Here's how the part is built. I have some questions about the finished solid (model axes, mm). A direction names the side the tool comes from. Round coordinates to 2 decimals unless told otherwise and drop trailing zeros. Put each result on its own line as item: value. Start each with the question number.
1. Suppose I cut it at A-A (x = 0). Count the separate pieces of the cut face and the enclosed holes in it, then the cut area to 3 significant figures.
2. For pin 1 (6 mm diameter, centred on x = -16, y = 17, fed in from -Z); pin 2 (1.5 mm diameter, centred on x = 1.5, z = -10, fed in from -Y); pin 3 (2.5 mm diameter, centred on x = -1.5, y = -0.5, fed in from -Z), each with a flat end and sliding along its axis, tell me the tip position at first contact or that it passes through.
3. We'd pull the mould along X, two halves only. Please class faces 4 (the face through (0, 0, 0)), 5 (the face through (-18.57, -0.65, -12.63)): +X half, -X half, draft (parallel to the pull), parting line (faces both ways), or undercut.
4. Which directions (+Z, -Z, +X, -X, +Y, -Y) give clear straight access to the entire face, cutting with the end or side of a thin tool? Please do faces 1 (the face through (-0.221, 19.686, -2.465)), 2 (the face through (0, -16, -5)), 3 (the face through (-11.547, -14.588, -1.479)).
5. I need wall thicknesses on probe 1 along Y at (x, z) = (8.5, -16); probe 2 along Y at (x, z) = (11, -2.25); probe 3 along Z at (x, y) = (-19, -9). Which ranges of each line are inside material? Lowest first, please. Write a range as from..to.
```python
from build123d import *

# Parameters (mm, degrees)
SKETCH_1_W                   = 25
SKETCH_1_H                   = 1
SKETCH_2_R                   = 22.55
EXTRUDE_1_DEPTH              = 10
HOLE_WIZARD_M3_1_D           = 3.4
HOLE_WIZARD_M3_1_DEPTH       = 11
HOLE_WIZARD_M3_1_CBORE_D     = 4.5
HOLE_WIZARD_M3_1_CBORE_DEPTH = 6
HOLE_WIZARD_1_D              = 8
HOLE_WIZARD_1_DEPTH          = 5
HOLE_WIZARD_1_CBORE_D        = 10.16
HOLE_WIZARD_1_CBORE_DEPTH    = 3
HOLE_WIZARD_M3_2_D           = 3.4
HOLE_WIZARD_M3_2_DEPTH       = 22
HOLE_WIZARD_M3_2_CBORE_D     = 6.1
HOLE_WIZARD_M3_2_CBORE_DEPTH = 3
CHAMFER_1_SIZE               = 1.05


with BuildPart() as part:
    # 草图1 → 旋转1 (revolve)
    with BuildSketch(Plane(origin=(0, 0, 0), x_dir=(1, 0, 0), z_dir=(0, 1, 0))):
        with Locations((12.5, 10.5)):
            Rectangle(SKETCH_1_W, SKETCH_1_H)
    revolve(axis=Axis((0, 0, -11), (0, 0, 1)))

    # 草图2 → 凸台-拉伸1 (add)
    with BuildSketch(Plane.XY.offset(-10)):
        Circle(SKETCH_2_R)
    extrude(amount=EXTRUDE_1_DEPTH)

    # 草图3 → 旋转2 (revolve)
    with BuildSketch(Plane(origin=(0, -14.722431864, 0), x_dir=(1, 0, 0), z_dir=(0, 1, 0))):
        Polygon((11.56, 22), (8.5, 22), (8.5, 11), (12.5, 11), (12.5, 12.5), (11.56, 12.5), align=None)
    revolve(axis=Axis((8.5, -14.722431864, -22), (0, 0, 1)))

    # 草图4 → 旋转3 (revolve)
    with BuildSketch(Plane(origin=(0, -14.722431864, 0), x_dir=(1, 0, 0), z_dir=(0, 1, 0))):
        Polygon((-5.44, 22), (-8.5, 22), (-8.5, 11), (-4.5, 11), (-4.5, 12.5), (-5.44, 12.5), align=None)
    revolve(axis=Axis((-8.5, -14.722431864, -22), (0, 0, 1)))

    # 草图5 → 旋转4 (revolve)
    with BuildSketch(Plane(origin=(0, 0, 0), x_dir=(1, 0, 0), z_dir=(0, 1, 0))):
        Polygon((-13.94, 22), (-17, 22), (-17, 11), (-13, 11), (-13, 12.5), (-13.94, 12.5), align=None)
    revolve(axis=Axis((-17, 0, -22), (0, 0, 1)))

    # 草图6 → 旋转5 (revolve)
    with BuildSketch(Plane(origin=(0, 14.722431864, 0), x_dir=(1, 0, 0), z_dir=(0, 1, 0))):
        Polygon((-5.44, 22), (-8.5, 22), (-8.5, 11), (-4.5, 11), (-4.5, 12.5), (-5.44, 12.5), align=None)
    revolve(axis=Axis((-8.5, 14.722431864, -22), (0, 0, 1)))

    # 草图7 → 旋转6 (revolve)
    with BuildSketch(Plane(origin=(0, 14.722431864, 0), x_dir=(1, 0, 0), z_dir=(0, 1, 0))):
        Polygon((11.56, 22), (8.5, 22), (8.5, 11), (12.5, 11), (12.5, 12.5), (11.56, 12.5), align=None)
    revolve(axis=Axis((8.5, 14.722431864, -22), (0, 0, 1)))

    # 草图8 → 旋转7 (revolve)
    with BuildSketch(Plane(origin=(0, 0, 0), x_dir=(1, 0, 0), z_dir=(0, 1, 0))):
        Polygon((20.06, 22), (17, 22), (17, 11), (21, 11), (21, 12.5), (20.06, 12.5), align=None)
    revolve(axis=Axis((17, 0, -22), (0, 0, 1)))

    # M3 六角头机械螺钉的柱形沉头孔1
    with Locations(Plane(origin=(0, 0, -11), x_dir=(-1, 0, 0), z_dir=(0, 0, -1))):
        with Locations((15.588457268, 9), (0, 18), (-15.588457268, 9), (-15.588457268, -9), (0, -18), (15.588457268, -9)):
            CounterBoreHole(HOLE_WIZARD_M3_1_D / 2, HOLE_WIZARD_M3_1_CBORE_D / 2, HOLE_WIZARD_M3_1_CBORE_DEPTH, depth=HOLE_WIZARD_M3_1_DEPTH)

    # 孔1
    with Locations(Plane(origin=(0, 0, -11), x_dir=(-1, 0, 0), z_dir=(0, 0, -1))):
        with Locations((0, 0)):
            CounterBoreHole(HOLE_WIZARD_1_D / 2, HOLE_WIZARD_1_CBORE_D / 2, HOLE_WIZARD_1_CBORE_DEPTH, depth=HOLE_WIZARD_1_DEPTH)

    # M3 六角头机械螺钉的柱形沉头孔2
    with Locations(Plane.XY):
        with Locations((8.5, -14.722431864), (-8.5, -14.722431864), (-17, 0), (-8.5, 14.722431864), (8.5, 14.722431864), (17, 0)):
            CounterBoreHole(HOLE_WIZARD_M3_2_D / 2, HOLE_WIZARD_M3_2_CBORE_D / 2, HOLE_WIZARD_M3_2_CBORE_DEPTH, depth=HOLE_WIZARD_M3_2_DEPTH)

    # 倒角1
    chamfer_1_edges = [part.edges().sort_by_distance(p)[0] for p in [
        (-22.55, 0, 0),
    ]]
    chamfer(chamfer_1_edges, length=CHAMFER_1_SIZE)


solid = part.part
```
Verdict:
1. separate pieces: 3
1. enclosed holes: 0
1. area: 365 mm^2
2. pin 1: stops at z = -11
2. pin 2: stops at y = -24.99
2. pin 3: stops at z = -6
3. face 4: draft
3. face 5: undercut
4. face 1: +Z, -Z
4. face 2: -Z
4. face 3: +Z
5. probe 1: y = -17.78..-16.42, -13.02..-11.66, 11.66..13.02, 16.42..17.78
5. probe 2: y = -19.69..-16.47, -12.98..12.98, 16.47..19.69
5. probe 3: z = -11..0
